from build123d import *

# Parameters (mm, degrees)
SKETCH2_R           = 25
BOSS_EXTRUDE1_DEPTH = 10
SKETCH3_R           = 6
CUT_EXTRUDE1_DEPTH  = 5
SKETCH4_R           = 10
CUT_EXTRUDE2_DEPTH  = 5


with BuildPart() as part:
    # Sketch2 → Boss-Extrude1 (new body)
    with BuildSketch(Plane.XY):
        Circle(SKETCH2_R)
    extrude(amount=BOSS_EXTRUDE1_DEPTH)

    # Sketch3 → Cut-Extrude1 (cut)
    with BuildSketch(Plane.XY.offset(10)):
        Circle(SKETCH3_R)
    extrude(amount=-CUT_EXTRUDE1_DEPTH, mode=Mode.SUBTRACT)

    # Sketch4 → Cut-Extrude2 (cut)
    with BuildSketch(Plane(origin=(0, 0, 0), x_dir=(-1, 0, 0), z_dir=(0, 0, -1))):
        Circle(SKETCH4_R)
    extrude(amount=-CUT_EXTRUDE2_DEPTH, mode=Mode.SUBTRACT)


solid = part.part
Read the model definition and answer for the solid it produces. Units are mm, in the model's axes. A direction names the side the tool comes from. Round coordinates to 2 decimals unless told otherwise and drop trailing zeros. Write each loop counter-clockwise with the first axis right and the second up, starting at its lowest first coordinate (ties: lowest second). Pieces come first, ordered by that corner, then holes. Notation, with made-up numbers: M 19,13.5 L 68,13.5 A16 cw 68,32.5 Z; hole C 17.25,75 d5. An arc over 180 degrees is marked long. Use a Markdown table: item, result.
1) A tool of negligible diameter and unlimited length cuts with its end or side. For faces 4 (the flat face through (0, -7, 5)), 5 (the cylindrical face through (-6, 0, 8)), from which of +Z, -Z, +X, -X, +Y, -Y can it reach the whole face along a straight path? Write none if from no direction.
Answers follow:
| item | result |
|---|---|
| face 4 | -Z |
| face 5 | +Z, -Z |
2) Flat-ended cylindrical pins translate along their axes: pin 1 (8 mm diameter, centred on x = 5, y = -17, fed in from -Z); pin 2 (4 mm diameter, centred on y = -17, z = 8.5, fed in from -X); pin 3 (1 mm diameter, centred on x = -18.5, z = 6, fed in from +Y); pin 4 (4 mm diameter, centred on y = -14, z = 7.5, fed in from -X). Find the tip coordinate at first contact, or state that the pin passes through.
Answers follow:
| item | result |
|---|---|
| pin 1 | stops at z = 0 |
| pin 2 | stops at x = -20 |
| pin 3 | stops at y = 17.35 |
| pin 4 | stops at x = -21.93 |
3) The part is cut by section C-C (z = 5.75). Write down the section's boundary in (x, y).
Answers follow:
| item | result |
|---|---|
| outline | C 0,0 d50; hole C 0,0 d12 |
4) The part is cut by section A-A (y = 0). Write down the section's boundary in (x, z), plus the area to 3 significant figures.
Answers follow:
| item | result |
|---|---|
| outline | M -25,0 L -10,0 L -10,5 L -6,5 L -6,10 L -25,10 Z; M 6,5 L 10,5 L 10,0 L 25,0 L 25,10 L 6,10 Z |
| area | 340 mm2 |
5) The part is cut by section B-B (x = -2). Write down the section's boundary in (y, z).
Answers follow:
| item | result |
|---|---|
| outline | M -24.92,0 L -9.8,0 L -9.8,5 L -5.66,5 L -5.66,10 L -24.92,10 Z; M 5.66,5 L 9.8,5 L 9.8,0 L 24.92,0 L 24.92,10 L 5.66,10 Z |
6) Straight lines are drawn through the part: line 1 along Y through (x, z) = (0, 9.75); line 2 along Y through (x, z) = (0, 3.55); line 3 along X through (y, z) = (5.5, 8.75). For each, find the intervals that lie inside material, in ascending order. Write a range as [from, to].
Answers follow:
| item | result |
|---|---|
| line 1 | y = [-25, -6], [6, 25] |
| line 2 | y = [-25, -10], [10, 25] |
| line 3 | x = [-24.39, -2.4], [2.4, 24.39] |
7) For a pull along X with two mould halves and no side action, classify faces 1 (the flat face through (5, -5, 10)), 2 (the cylindrical face through (23.846, 7.509, 4.93)), 3 (the cylindrical face through (2.17, -9.76, 2.46)) as pulls with the +X half, pulls with the -X half, needs draft (parallel to the pull), parting line crosses it, or undercut.
Answers follow:
| item | result |
|---|---|
| face 1 | needs draft |
| face 2 | parting line crosses it |
| face 3 | undercut |
8) The part is cut by section D-D (y = 15). Write down the section's boundary in (x, z).
Answers follow:
| item | result |
|---|---|
| outline | M -20,0 L 20,0 L 20,10 L -20,10 Z |
